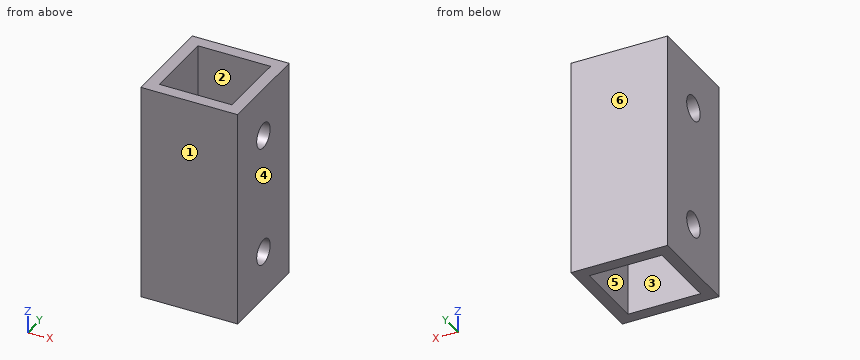
Autodesk Inventor part; units mm, degrees
ref_plane "YZ Plane" through (0, 0, 0) normal (1, 0, 0) x (0, 1, 0)
ref_plane "XZ Plane" through (0, 0, 0) normal (0, 1, 0) x (-1, 0, 0)
ref_plane "XY Plane" through (0, 0, 0) normal (0, 0, 1) x (1, 0, 0)
sketch "Sketch1" plane through (0, 0, 0) normal (0, 0, 1) x (1, 0, 0)
  line L0 (0, 0) -> (25.4, 0)
  line L1 (25.4, 0) -> (25.4, 25.4)
  line L2 (25.4, 25.4) -> (0, 25.4)
  line L3 (0, 25.4) -> (0, 0)
  line L4 (3.175, 22.225) -> (22.225, 22.225)
  line L5 (22.225, 22.225) -> (22.225, 3.175)
  line L6 (22.225, 3.175) -> (3.175, 3.175)
  line L7 (3.175, 3.175) -> (3.175, 22.225)
  dimension "d0" = 25.4
  dimension "d1" = 25.4
  dimension "d2" = 3.175
extrude "Extrusion1" add sketch "Sketch1" along normal blind 57.15
sketch "Sketch2" plane through (25.4, 0, 0) normal (1, 0, 0) x (0, 0, -1)
  line L0 (0, 0) -> (0, 25.4)
  line L1 (-57.15, 0) -> (-57.15, 25.4)
  circle A0 centre (-12.7, 12.7) radius 3.302
  circle A1 centre (-44.45, 12.7) radius 3.302
  line L2 (-57.15, 12.7) -> (0, 12.7) construction
  dimension "d5" = 31.75
  dimension "d7" = 12.7
  dimension "d8" = 6.604
extrude "Extrusion2" cut sketch "Sketch2" against normal through all
properties part number "Chassis Part 11 (26x28)" material "Aluminum 6061"
Check sheet for the modelled part. Datum: model origin and axes. Units: mm. Face numbers are marked on the shaded views. A direction names the side the tool comes from. Coordinates: 2 decimals unless noted, no trailing zeros. Write each loop counter-clockwise with the first axis right and the second up, starting at its lowest first coordinate (ties: lowest second). Pieces come first, ordered by that corner, then holes. Notation, with made-up numbers: (-13, 74) - (23, 74) arc R26 cw to (23, 89) - close; hole circle Ø9 at (18, 46.5). An arc over 180 degrees is marked (long way). One line per question, with ' | ' between items.
Item 1: Mould release check, pull along X, two halves, no side actions. Record for the marked faces 1, 2, 3 and 4: pulls with the +X half, pulls with the -X half, needs draft (parallel to the pull), parting line crosses it, or undercut.
Determined:
face 1: needs draft | face 2: undercut | face 3: undercut | face 4: pulls with the +X half
Item 2: Sectioned sample at D-D on z = 32. Record the boundary of the cut face in (x, y) (3 decimals).
Determined:
outline: (0, 0) - (25.4, 0) - (25.4, 25.4) - (0, 25.4) - close; hole (3.175, 3.175) - (22.225, 3.175) - (22.225, 22.225) - (3.175, 22.225) - close
Item 3: Access from +Z, -Z, +X, -X, +Y, -Y to the whole of each face (thin tool, end or side, straight path). Record for the marked faces 5 and 6.
Determined:
face 5: +Z, -Z | face 6: +Z, -Z, +X, -X, +Y
Item 4: Sectioned sample at C-C on y = 12.7. Record the boundary of the cut face in (x, z) (3 decimals).
Determined:
outline: (0, 0) - (3.175, 0) - (3.175, 9.398) - (0, 9.398) - close; (0, 16.002) - (3.175, 16.002) - (3.175, 41.148) - (0, 41.148) - close; (0, 47.752) - (3.175, 47.752) - (3.175, 57.15) - (0, 57.15) - close; (22.225, 0) - (25.4, 0) - (25.4, 9.398) - (22.225, 9.398) - close; (22.225, 16.002) - (25.4, 16.002) - (25.4, 41.148) - (22.225, 41.148) - close; (22.225, 47.752) - (25.4, 47.752) - (25.4, 57.15) - (22.225, 57.15) - close
Item 5: Sectioned sample at A-A on x = 15.5. Record the boundary of the cut face in (y, z) (3 decimals).
Determined:
outline: (0, 0) - (3.175, 0) - (3.175, 57.15) - (0, 57.15) - close; (22.225, 0) - (25.4, 0) - (25.4, 57.15) - (22.225, 57.15) - close
Item 6: Sectioned sample at B-B on z = 12.7. Record the boundary of the cut face in (x, y) (3 decimals), plus the area to 3 significant figures.
Determined:
outline: (0, 0) - (25.4, 0) - (25.4, 9.398) - (22.225, 9.398) - (22.225, 3.175) - (3.175, 3.175) - (3.175, 9.398) - (0, 9.398) - close; (0, 16.002) - (3.175, 16.002) - (3.175, 22.225) - (22.225, 22.225) - (22.225, 16.002) - (25.4, 16.002) - (25.4, 25.4) - (0, 25.4) - close | area: 240 mm2
Item 7: Gauge pin test, flat end, axial feed: P1, Ø6, axis at x = 11.5, z = 26.5, coming from the -Y side. Record the tip position at first contact, or that the pin passes through.
Determined:
P1: stops at y = 0
Item 8: Thickness scan on line 1 (X direction, y = 17.5, z = 49) (3 decimals); line 2 (Y direction, x = 1, z = 44.45). Record the ranges inside material, lowest first. Write a range as [from, to].
Determined:
line 1: x = [0, 3.175], [22.225, 25.4] | line 2: y = [0, 9.4], [16, 25.4]
